The model under review builds one solid part; all positions refer to its coordinate system, in mm. A direction names the side the tool comes from. Give positions to 0.01 mm unless a question says otherwise; leave off trailing zeros. Order: outer loops, then holes, each group sorted by start corner. A loop starts at its lowest first (then second) coordinate and runs counter-clockwise, first axis right, second up. Notation, with made-up numbers: (74.5, -14) -> (103.5, -14) arc R19 ccw to (103.5, -7) -> close; hole circle Ø4 at (-19.75, -30). An arc over 180 degrees is marked (long way). Use one line per item in the form item = value.
```python
from build123d import *

# Parameters (mm, degrees)
SKETCH1_W           = 68
SKETCH1_H           = 110
SKETCH1_R           = 2.1
SKETCH1_R_2         = 4.05
BOSS_EXTRUDE1_DEPTH = 7.7
SKETCH2_R           = 6.304633146
SKETCH2_R_2         = 7.334333348
SKETCH2_R_3         = 8.114040952
SKETCH2_R_4         = 11.073656437
BOSS_EXTRUDE2_DEPTH = 5
SKETCH3_R           = 4.05
CUT_EXTRUDE1_DEPTH  = 4


with BuildPart() as part:
    # Sketch1 → Boss-Extrude1 (new body)
    with BuildSketch(Plane.XY):
        Rectangle(SKETCH1_W, SKETCH1_H)
        with Locations((20, 45)):
            Circle(SKETCH1_R, mode=Mode.SUBTRACT)
        with Locations((-20, 45)):
            Circle(SKETCH1_R, mode=Mode.SUBTRACT)
        with Locations((20, -45)):
            Circle(SKETCH1_R, mode=Mode.SUBTRACT)
        with Locations((-20, -45)):
            Circle(SKETCH1_R, mode=Mode.SUBTRACT)
        with Locations((21.650635095, -12.5)):
            Circle(SKETCH1_R_2, mode=Mode.SUBTRACT)
        with Locations((0, 25)):
            Circle(SKETCH1_R_2, mode=Mode.SUBTRACT)
        with Locations((-21.650635095, -12.5)):
            Circle(SKETCH1_R_2, mode=Mode.SUBTRACT)
        with Locations((0, -36.95)):
            Circle(SKETCH1_R_2, mode=Mode.SUBTRACT)
    extrude(amount=BOSS_EXTRUDE1_DEPTH)

    # Sketch2 → Boss-Extrude2 (add)
    with BuildSketch(Plane(origin=(0, 0, 0), x_dir=(-1, 0, 0), z_dir=(0, 0, -1))):
        with Locations((-21.650635095, -12.5)):
            Circle(SKETCH2_R)
        with Locations((0, 25)):
            Circle(SKETCH2_R_2)
        with Locations((21.650635095, -12.5)):
            Circle(SKETCH2_R_3)
        with Locations((0, -36.95)):
            Circle(SKETCH2_R_4)
    extrude(amount=-BOSS_EXTRUDE2_DEPTH)

    # Sketch3 → Cut-Extrude1 (cut)
    with BuildSketch(Plane(origin=(0, 0, 7.7), x_dir=(-1, 0, 0), z_dir=(0, 0, -1))):
        with Locations((-20, 45)):
            Circle(SKETCH3_R)
        with Locations((20, 45)):
            Circle(SKETCH3_R)
        with Locations((-20, -45)):
            Circle(SKETCH3_R)
        with Locations((20, -45)):
            Circle(SKETCH3_R)
    extrude(amount=CUT_EXTRUDE1_DEPTH, mode=Mode.SUBTRACT)


solid = part.part
```
1. Add section C-C on x = 0. Give the boundary of the cut face in (y, z).
Values:
outline = (-55, 0) -> (55, 0) -> (55, 7.7) -> (29.05, 7.7) -> (29.05, 5) -> (20.95, 5) -> (20.95, 7.7) -> (-32.9, 7.7) -> (-32.9, 5) -> (-41, 5) -> (-41, 7.7) -> (-55, 7.7) -> close
2. The part is to be moulded in two halves that separate along Y. For faces 3 (the face through (0, -55, 4)), 4 (the face through (0, 55, 4)), 5 (the face through (-0.527, -32.934, 6.331)), say which applies: +Y half, -Y half, draft (parallel to the pull), parting line (faces both ways), or undercut.
Values:
face_3 = -Y half
face_4 = +Y half
face_5 = undercut
3. Add section A-A on x = -19.5. Give the boundary of the cut face in (y, z).
Values:
outline = (-55, 0) -> (-47.04, 0) -> (-47.04, 3.7) -> (-49.02, 3.7) -> (-49.02, 7.7) -> (-55, 7.7) -> close; (-42.96, 0) -> (42.96, 0) -> (42.96, 3.7) -> (40.98, 3.7) -> (40.98, 7.7) -> (-9.07, 7.7) -> (-9.07, 5) -> (-15.93, 5) -> (-15.93, 7.7) -> (-40.98, 7.7) -> (-40.98, 3.7) -> (-42.96, 3.7) -> close; (47.04, 0) -> (55, 0) -> (55, 7.7) -> (49.02, 7.7) -> (49.02, 3.7) -> (47.04, 3.7) -> close
4. Add section D-D on y = -36.95. Give the boundary of the cut face in (x, z), then the cut area to 3 significant figures.
Values:
outline = (-34, 0) -> (34, 0) -> (34, 7.7) -> (4.05, 7.7) -> (4.05, 5) -> (-4.05, 5) -> (-4.05, 7.7) -> (-34, 7.7) -> close
area = 502 mm^2
5. For L1, parallel to X at y = 45, z = 1.8; L2, parallel to X at y = -12.5, z = 6.95; L3, parallel to Y at x = 0, z = 6.95, list the stretches that pass through material, from the lowest coordinate up.
Values:
L1 = -34 to -22.1, -17.9 to 17.9, 22.1 to 34
L2 = -34 to -25.7, -17.6 to 17.6, 25.7 to 34
L3 = -55 to -41, -32.9 to 20.95, 29.05 to 55
6. Add section B-B on y = -12.5. Give the boundary of the cut face in (x, z).
Values:
outline = (-34, 0) -> (34, 0) -> (34, 7.7) -> (25.7, 7.7) -> (25.7, 5) -> (17.6, 5) -> (17.6, 7.7) -> (-17.6, 7.7) -> (-17.6, 5) -> (-25.7, 5) -> (-25.7, 7.7) -> (-34, 7.7) -> close
7. Tool access review of faces 1 (the face through (0, -37, 5)), 2 (the face through (-34, -1, 4)): name each direction out of +Z, -Z, +X, -X, +Y, -Y from which nothing blocks a thin tool from reaching the whole face with its end or side.
Values:
face_1 = +Z
face_2 = +Z, -Z, -X, +Y, -Y
8. For pin 1 Ø4 at (x, y) = (-18.5, -44) entering from +Z; pin 2 Ø2.5 at (x, y) = (21.5, -13) entering from +Z, all flat-tipped, find the tip position at first contact; note any pin that passes through.
Values:
pin_1 = 3.7
pin_2 = 5
